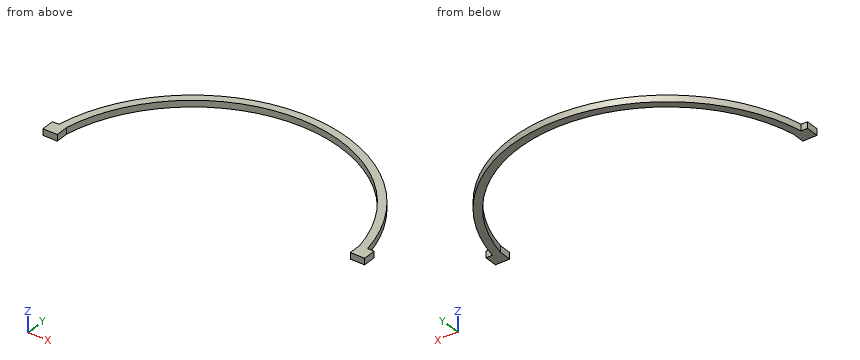
from build123d import *

# Parameters (mm, degrees)
BOSS_EXTRUDE1_DEPTH = 3.175
SKETCH2_W           = 7.051872993
SKETCH2_H           = 3.175
BOSS_EXTRUDE2_DEPTH = 6.35


with BuildPart() as part:
    # Sketch1 → Boss-Extrude1 (new body)
    with BuildSketch(Plane.XY):
        with BuildLine():
            Line((-76.2, 0), (-72.323127007, 0))
            ThreePointArc((-72.323127007, 0), (0, 59.69), (72.323127007, 0))
            Line((72.323127007, 0), (76.2, 0))
            ThreePointArc((76.2, 0), (0, 63.5), (-76.2, 0))
        make_face()
    extrude(amount=BOSS_EXTRUDE1_DEPTH)

    # Sketch2 → Boss-Extrude2 (add)
    with BuildSketch(Plane.XZ):
        with Locations((75.849063504, 1.5875)):
            Rectangle(SKETCH2_W, SKETCH2_H)
        with Locations((-75.849063504, 1.5875)):
            Rectangle(SKETCH2_W, SKETCH2_H)
    extrude(amount=BOSS_EXTRUDE2_DEPTH)


solid = part.part
Could you check a few things on this model? Use its own coordinates, in mm. Give positions to 0.01 mm unless a question says otherwise; leave off trailing zeros. Order: outer loops, then holes, each group sorted by start corner. A loop starts at its lowest first (then second) coordinate and runs counter-clockwise, first axis right, second up.
Item 1: I need wall thicknesses on line 1 (X direction, y = 40, z = 0.55); line 2 (X direction, y = -2, z = 0.2) (3 decimals); line 3 (Y direction, x = 67, z = 0.9). Which ranges of each line are inside material? Lowest first, please.
Item 2: If we section it at B-B, the plane z = 2: Write out the boundary of the cut face in (x, y) (3 decimals).
Item 3: If we section it at C-C, the plane y = 5: Write out the boundary of the cut face in (x, z) (3 decimals), plus the area to 3 significant figures.
Item 4: If we section it at A-A, the plane y = 32: Write out the boundary of the cut face in (x, z) (3 decimals).
Item 5: If we section it at D-D, the plane x = 3.5: Write out the boundary of the cut face in (y, z) (3 decimals), plus the area to 3 significant figures.
Item 6: I'm going to push flat-ended pins straight in: pin 1 (1 mm diameter, centred on y = 47, z = 2.5, fed in from +X) (3 decimals); pin 2 (1 mm diameter, centred on x = 77.5, z = 2, fed in from +Y). Where does each tip first touch, or does it pass through?
Values:
1. line 1: x = -55.58 to -50.13, 50.13 to 55.58
1. line 2: x = -79.375 to -72.323, 72.323 to 79.375
1. line 3: y = 16.64 to 24.92
2. outline: (-79.375, -6.35) - (-72.323, -6.35) - (-72.323, 0) arc R73.66 cw to (72.323, 0) - (72.323, -6.35) - (79.375, -6.35) - (79.375, 0) - (76.2, 0) arc R77.47 ccw to (-76.2, 0) - (-79.375, 0) - close
3. outline: (-75.112, 0) - (-71.175, 0) - (-71.175, 3.175) - (-75.112, 3.175) - close; (71.175, 0) - (75.112, 0) - (75.112, 3.175) - (71.175, 3.175) - close
3. area: 25.0 mm2
4. outline: (-62.357, 0) - (-57.555, 0) - (-57.555, 3.175) - (-62.357, 3.175) - close; (57.555, 0) - (62.357, 0) - (62.357, 3.175) - (57.555, 3.175) - close
5. outline: (59.607, 0) - (63.421, 0) - (63.421, 3.175) - (59.607, 3.175) - close
5. area: 12.1 mm2
6. pin 1: stops at x = 48.425
6. pin 2: stops at y = 0
